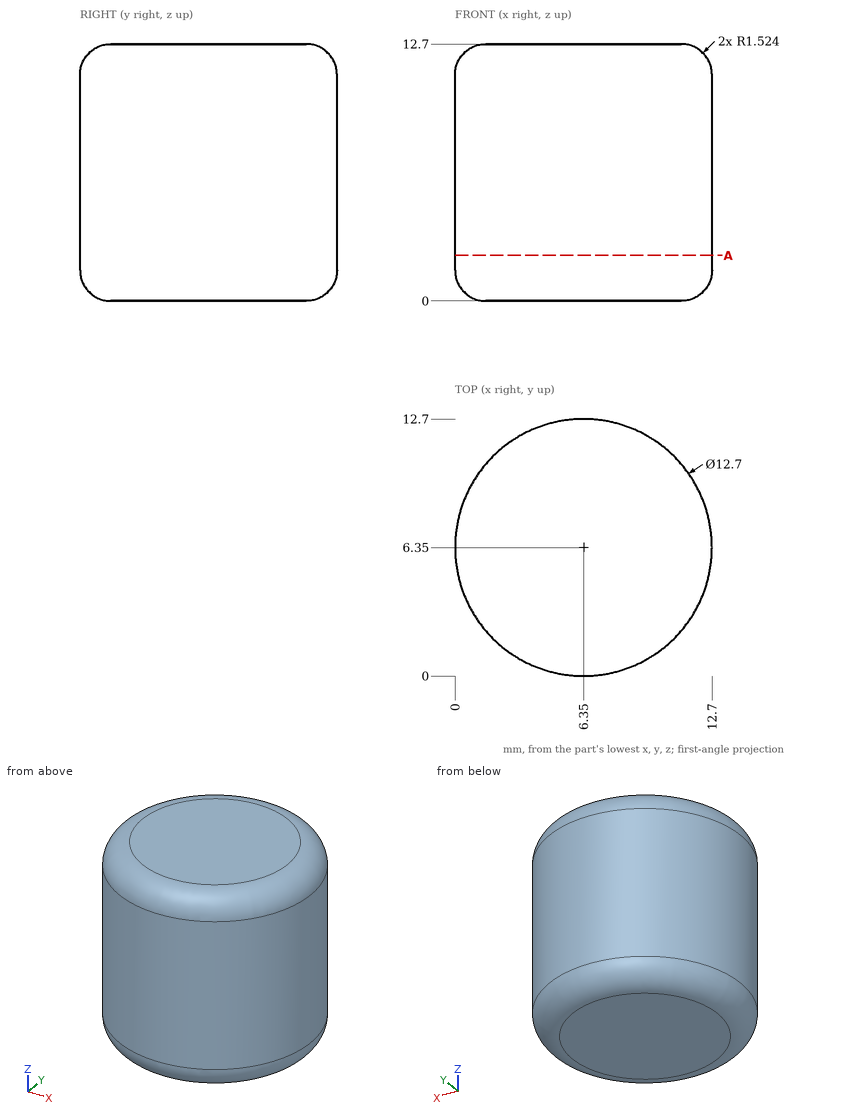
Print and shaded views of the part. All mm, measured from the part's lowest x, y and z. Coordinates: 2 decimals unless noted, no trailing zeros. Loops run counter-clockwise (first coordinate to the right, second up) from the corner with the lowest first, then second, coordinate; pieces in that order, holes last. Notation, with made-up numbers: M 17,11.25 L 55,11.25 A13 cw 55,34.25 Z; hole C 41.5,7 d10. An arc over 180 degrees is marked long. Use a Markdown table: item, result. Add a question column.
Q1. Pin check, flat tips, straight feed: P1, Ø6, axis at x = 10, z = 2.5, coming from the -Y side; P2, Ø2, axis at x = 3.5, z = 4.5, coming from the -Y side; P3, Ø1, axis at y = 4, z = 2.5, coming from the +X side. Stop position of each tip, or through.
Q2. Probe L1, parallel to X at y = 6.25, z = 10.5; L2, parallel to Y at x = 11.5, z = 10.25; L3, parallel to Y at x = 9.25, z = 10.5. List the from-to ranges inside material, lowest first.
Q3. Cut at A-A (z = 2.25). Write the cut outline in (x, y).
Worked out:
| question | item | result |
|---|---|---|
| 1 | P1 | stops at y = 0.03 |
| 1 | P2 | stops at y = 0.28 |
| 1 | P3 | stops at x = 12.42 |
| 2 | L1 | x = 0 to 12.7 |
| 2 | L2 | y = 2.64 to 10.06 |
| 2 | L3 | y = 0.7 to 12 |
| 3 | outline | C 6.35,6.35 d12.7 |
